Model file for the job. Use its own axes, mm. Face numbers are marked on the shaded views. A direction names the side the tool comes from. Round coordinates to 2 decimals unless told otherwise and drop trailing zeros. Order: outer loops, then holes, each group sorted by start corner. A loop starts at its lowest first (then second) coordinate and runs counter-clockwise, first axis right, second up. Notation, with made-up numbers: (-8, 33) -> (39, 33) arc R10 ccw to (39, 50) -> close; hole circle Ø4 at (87.5, -12). An arc over 180 degrees is marked (long way). Answer as CSV lines item,"result".
```python
from build123d import *

# Parameters (mm, degrees)
SKETCH1_R                   = 18.288
BOSS_EXTRUDE1_DEPTH         = 19.05
SKETCH3_R                   = 13.208
CUT_EXTRUDE1_DEPTH          = 33.121712096
SKETCH15_W                  = 19.05
SKETCH15_H                  = 17.526
BOSS_EXTRUDE3_DEPTH         = 15.24
SKETCH16_W                  = 11.43
SKETCH16_H                  = 5.842
CUT_EXTRUDE4_DEPTH          = 39.82462909
CHAMFER1_SIZE               = 8.129699408
CHAMFER1_SIZE_2             = 5.08
F_1_4_CLEARANCE_HOLE1_D     = 6.7564
F_1_4_CLEARANCE_HOLE1_DEPTH = 3.448428068
SKETCH19_R                  = 18.288
SKETCH19_R_2                = 13.208
CUT_EXTRUDE5_DEPTH          = 0.762
CUT_EXTRUDE6_START          = -2.54
SKETCH20_R                  = 18.288
CUT_EXTRUDE6_DEPTH          = 2.54
SKETCH21_R                  = 18.288
CUT_EXTRUDE7_DEPTH          = 7.493
SKETCH22_W                  = 19.05
SKETCH22_H                  = 4.191
CUT_EXTRUDE8_DEPTH          = 42.148
SKETCH24_R                  = 14.478
CUT_EXTRUDE10_DEPTH         = 5.334
SKETCH25_W                  = 8.255
SKETCH25_H                  = 5.08
BOSS_EXTRUDE4_DEPTH         = 15.24
F_4_CLEARANCE_HOLE1_D       = 3.4544
SKETCH28_W                  = 6.858
SKETCH28_H                  = 2.794
CUT_EXTRUDE11_DEPTH         = 43.003222079
MIRROR3_COPY_1_SKETCH_W     = 6.858
MIRROR3_COPY_1_SKETCH_H     = 2.794
MIRROR3_COPY_1_DEPTH        = 43.003222079
SKETCH29_W                  = 78.170578527
SKETCH29_H                  = 29.425688311
CUT_EXTRUDE12_DEPTH         = 35.306
CHAMFER2_SIZE               = 1.27


# Some blends are built 0.0001 mm under size
with BuildPart() as part:
    # Sketch1 → Boss-Extrude1 (new body)
    with BuildSketch(Plane.XY):
        with Locations(Location((0, 0, 0), (0, 0, 180))):
            Circle(SKETCH1_R)
    extrude(amount=BOSS_EXTRUDE1_DEPTH)

    # Sketch3 → Cut-Extrude1 (cut, through all)
    with BuildSketch(Plane.XY.offset(19.05)):
        Circle(SKETCH3_R)
    extrude(amount=-CUT_EXTRUDE1_DEPTH, mode=Mode.SUBTRACT)

    # Sketch15 → Boss-Extrude3 (add)
    with BuildSketch(Plane(origin=(0, -13.716, 0), x_dir=(1, 0, 0), z_dir=(0, 1, 0))):
        with Locations((0, -9.525)):
            Rectangle(SKETCH15_W, SKETCH15_H)
    extrude(amount=-BOSS_EXTRUDE3_DEPTH)

    # Sketch16 → Cut-Extrude4 (cut, through all)
    with BuildSketch(Plane.XY.offset(18.288)):
        with Locations((0, -22.586571932)):
            Rectangle(SKETCH16_W, SKETCH16_H)
    extrude(amount=-CUT_EXTRUDE4_DEPTH, mode=Mode.SUBTRACT)

    # Chamfer1
    # the kernel refuses this chamfer: 8.129699408, 5.08 mm, written as the material it takes off along each edge
    with BuildSketch(Plane(origin=(-30.543101737, -28.956, 0.762), x_dir=(0, 0.9997899140358644, -0.020497019104217945), z_dir=(1, 0, 0))) as chamfer1_piece_1:
        Polygon((CHAMFER1_SIZE * 0.999789913978, CHAMFER1_SIZE * 0.020497019103), (-CHAMFER1_SIZE_2 * 0.0204970191042, CHAMFER1_SIZE_2 * 0.999789914036), (0, 0), align=None)
    extrude(amount=61.086203475, mode=Mode.SUBTRACT)

    # 1/4 Clearance Hole1
    with Locations(Plane(origin=(0, -28.956, 0), x_dir=(-1, 0, 0), z_dir=(0, -1, 0))):
        with Locations((0, -12.021417661)):
            Hole(F_1_4_CLEARANCE_HOLE1_D / 2, depth=F_1_4_CLEARANCE_HOLE1_DEPTH)

    # Sketch19 → Cut-Extrude5 (cut)
    with BuildSketch(Plane.XY.offset(19.05)):
        with Locations(Location((0, 0, 0), (0, 0, 238.611833536))):
            Circle(SKETCH19_R)
        Circle(SKETCH19_R_2, mode=Mode.SUBTRACT)
    extrude(amount=-CUT_EXTRUDE5_DEPTH, mode=Mode.SUBTRACT)

    # Sketch20 → Cut-Extrude6 (cut)
    with BuildSketch(Plane.XY.offset(18.288).offset(CUT_EXTRUDE6_START)):
        with Locations(Location((0, 0, 0), (0, 0, 238.611833536))):
            Circle(SKETCH20_R)
    extrude(amount=CUT_EXTRUDE6_DEPTH, mode=Mode.SUBTRACT)

    # Sketch21 → Cut-Extrude7 (cut)
    with BuildSketch(Plane(origin=(0, 0, 0), x_dir=(-1, 0, 0), z_dir=(0, 0, -1))):
        Circle(SKETCH21_R)
    extrude(amount=-CUT_EXTRUDE7_DEPTH, mode=Mode.SUBTRACT)

    # Sketch22 → Cut-Extrude8 (cut, through all)
    with BuildSketch(Plane(origin=(0, -13.716, 0), x_dir=(1, 0, 0), z_dir=(0, 1, 0))):
        with Locations((0, -2.8575)):
            Rectangle(SKETCH22_W, SKETCH22_H)
    extrude(amount=-CUT_EXTRUDE8_DEPTH, mode=Mode.SUBTRACT)

    # Sketch24 → Cut-Extrude10 (cut)
    with BuildSketch(Plane.XY.offset(13.843)):
        Circle(SKETCH24_R)
    extrude(amount=-CUT_EXTRUDE10_DEPTH, mode=Mode.SUBTRACT)

    # Sketch25 → Boss-Extrude4 (add)
    with BuildSketch(Plane(origin=(13.208, 0, 0), x_dir=(0, 0, -1), z_dir=(1, 0, 0))):
        with Locations((-11.6205, 8.89)):
            Rectangle(SKETCH25_W, SKETCH25_H)
        with Locations((-11.6205, -8.89)):
            Rectangle(SKETCH25_W, SKETCH25_H)
    boss_extrude4 = extrude(amount=BOSS_EXTRUDE4_DEPTH)

    # #4 Clearance Hole1 (through all)
    with Locations(Plane(origin=(0, -11.43, 0), x_dir=(-1, 0, 0), z_dir=(0, -1, 0))):
        with Locations((-23.368, -11.6205)):
            f_4_clearance_hole1 = Hole(F_4_CLEARANCE_HOLE1_D / 2)

    # Sketch28 → Cut-Extrude11 (cut, through all)
    with BuildSketch(Plane.XY.offset(15.748)):
        with Locations((23.368, -8.89)):
            Rectangle(SKETCH28_W, SKETCH28_H)
    cut_extrude11 = extrude(amount=-CUT_EXTRUDE11_DEPTH, mode=Mode.SUBTRACT)

    # Mirror2: Cut-Extrude11 across plane
    add(cut_extrude11.mirror(Plane.ZX), mode=Mode.SUBTRACT)

    # Mirror3: Boss-Extrude4, #4 Clearance Hole1, Cut-Extrude11 across plane
    add(boss_extrude4.mirror(Plane(origin=(0, 0, 0), x_dir=(0, 0, 1), z_dir=(1, 0, 0))))
    add(f_4_clearance_hole1.mirror(Plane(origin=(0, 0, 0), x_dir=(0, 0, 1), z_dir=(1, 0, 0))), mode=Mode.SUBTRACT)
    add(cut_extrude11.mirror(Plane(origin=(0, 0, 0), x_dir=(0, 0, 1), z_dir=(1, 0, 0))), mode=Mode.SUBTRACT)

    # Mirror3 copy 1 sketch → Mirror3 copy 1 (cut, through all)
    with BuildSketch(Plane(origin=(0, 0, 15.748), x_dir=(-1, 0, 0), z_dir=(0, 0, 1))):
        with Locations((23.368, -8.89)):
            Rectangle(MIRROR3_COPY_1_SKETCH_W, MIRROR3_COPY_1_SKETCH_H)
    extrude(amount=-MIRROR3_COPY_1_DEPTH, mode=Mode.SUBTRACT)

    # Sketch29 → Cut-Extrude12 (cut)
    with BuildSketch(Plane.XZ.offset(28.956)):
        with Locations((-0.790643495, 9.076690496)):
            Rectangle(SKETCH29_W, SKETCH29_H)
    extrude(amount=-CUT_EXTRUDE12_DEPTH, mode=Mode.SUBTRACT)

    # Chamfer2
    chamfer2_edges = [part.edges().sort_by_distance(p)[0] for p in [
        (0, 14.478, 8.509),
        (0, 14.478, 13.843),
    ]]
    chamfer(chamfer2_edges, length=CHAMFER2_SIZE - 0.0001)  # a hair under: the kernel refuses the full size


solid = part.part
```
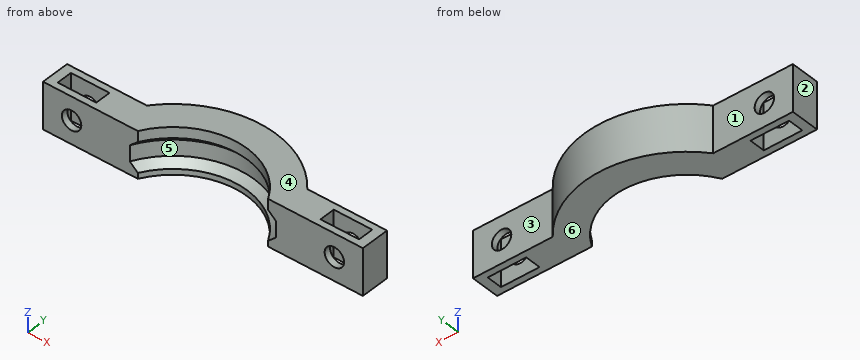
Q1. Flat gauge pins, fed straight in: pin 1 (4 mm diameter, centred on x = -20, z = 11, fed in from +Y); pin 2 (3 mm diameter, centred on x = -23.37, z = 11.62, fed in from +Y). Where does each tip first touch, or does it go through?
Checks:
pin 1,"y = 11.43"
pin 2,"through"
Q2. Wall check: L1, parallel to X at y = 8.5, z = 9; L2, parallel to Y at x = 22.5, z = 14.5; L3, parallel to X at y = 8.25, z = 10.25. Give the ranges that are in metal, low to high. Write a range as [from, to].
Checks:
L1,"[-28.45, -26.8], [-19.94, -10.74], [10.74, 19.94], [26.8, 28.45]"
L2,"[6.35, 7.49], [10.29, 11.43]"
L3,"[-28.45, -26.8], [-19.94, -11.9], [11.9, 19.94], [26.8, 28.45]"
Q3. Saw through at C-C (y = 9.25). State how many separate pieces and enclosed holes the cut face has, plus the area to 3 significant figures.
Checks:
separate pieces,"4"
enclosed holes,"0"
area,"187 mm²"
Q4. Tool access for the marked faces 1 and 2: list every direction of +Z, -Z, +X, -X, +Y, -Y with a clear straight run to the whole face (end or side of a thin tool).
Checks:
face 1,"+Z, -Z, -X, +Y"
face 2,"+Z, -Z, -X, +Y, -Y"
Q5. Saw through at B-B (x = 16). Write the cut outline in (y, z), plus the area to 3 significant figures.
Checks:
outline,"(6.35, 7.49) -> (11.43, 7.49) -> (11.43, 15.75) -> (6.35, 15.75) -> close"
area,"41.9 mm²"
Q6. Saw through at D-D (y = 16). Write the cut outline in (x, z).
Checks:
outline,"(-8.86, 7.49) -> (8.86, 7.49) -> (8.86, 15.75) -> (-8.86, 15.75) -> close"
Q7. Saw through at A-A (z = 15.25). Write the cut outline in (x, y), plus the area to 3 significant figures.
Checks:
outline,"(-28.45, 6.35) -> (-11.58, 6.35) arc R13.21 cw to (11.58, 6.35) -> (28.45, 6.35) -> (28.45, 11.43) -> (14.28, 11.43) arc R18.29 ccw to (-14.28, 11.43) -> (-28.45, 11.43) -> close; hole (-26.8, 7.49) -> (-19.94, 7.49) -> (-19.94, 10.29) -> (-26.8, 10.29) -> close; hole (19.94, 7.49) -> (26.8, 7.49) -> (26.8, 10.29) -> (19.94, 10.29) -> close"
area,"274 mm²"
Q8. Mould opens along Z. For the marked faces 3, 4, 5 and 6 say: +Z half, -Z half, draft (parallel to the pull), parting line (faces both ways), or undercut.
Checks:
face 3,"draft"
face 4,"+Z half"
face 5,"undercut"
face 6,"-Z half"
